Autodesk Inventor part; units mm, degrees
ref_plane "Start plane" through (0, 0, 0) normal (0, 0, 1) x (1, 0, 0)
ref_plane "End plane" through (0, 0, 796) normal (0, 0, 1) x (1, 0, 0)
ref_plane "YZ Plane" through (0, 0, 0) normal (1, 0, 0) x (0, 1, 0)
ref_plane "Start plane" through (0, 0, 0) normal (0, 0, 1) x (1, 0, 0)
ref_plane "End plane" through (0, 0, 796) normal (0, 0, 1) x (1, 0, 0)
sketch "Sketch" plane through (0, 0, 0) normal (0, 0, 1) x (1, 0, 0)
  line L0 (-10, -16) -> (-10, 16)
  line L1 (-6, 20) -> (6, 20)
  line L2 (10, 16) -> (10, -16)
  line L3 (6, -20) -> (-6, -20)
  arc A0 (-10, -16) -> (-6, -20) centre (-6, -16) ccw
  arc A1 (10, 16) -> (6, 20) centre (6, 16) ccw
  arc A2 (-6, 20) -> (-10, 16) centre (-6, 16) ccw
  arc A3 (6, -20) -> (10, -16) centre (6, -16) ccw
  arc A4 (-6, 18) -> (-8, 16) centre (-6, 16) ccw
  line L4 (-6, 18) -> (6, 18)
  arc A5 (8, 16) -> (6, 18) centre (6, 16) ccw
  line L5 (8, 16) -> (8, -16)
  arc A6 (6, -18) -> (8, -16) centre (6, -16) ccw
  line L6 (6, -18) -> (-6, -18)
  arc A7 (-8, -16) -> (-6, -18) centre (-6, -16) ccw
  line L7 (-8, -16) -> (-8, 16)
  line L8 (0, 29.1598) -> (0, -29.1598) construction
  line L9 (-15.1598, 0) -> (15.1598, 0) construction
  dimension "d7" = 4
  dimension "d9" = 20
  dimension "d11" = 40
  dimension "d12" = 2
  dimension "d15" = 10
  dimension "d16" = 20
extrude "Body" add sketch "Sketch" along normal up to surface (796 mm away) from surface at 0
sketch "Sketch3" plane through (0, 0, 0) normal (0, 0, 1) x (1, 0, 0)
  line L0 (0, 0) -> (10, 0)
ref_plane "Work Plane3" through (0, 0, 0) normal (0, -1, 0) x (1, 0, 0)
sketch "Sketch5" plane through (-6, -20, 0) normal (0, -1, 0) x (1, 0, 0)
  line L0 (-4, 0) -> (-4, 796)
  line L1 (-4, 796) -> (0, 796)
  line L2 (12, 796) -> (0, 796)
  line L3 (12, 796) -> (16, 796)
  line L4 (16, 0) -> (16, 796)
  line L5 (16, 796) -> (-4, 782.7623)
  point P0 (6, 0)
  dimension "d19" = 33.5
extrude "Extrusion2" cut sketch "Sketch5" against normal through all
sketch "Sketch4" plane through (0, 0, 0) normal (0, -1, 0) x (1, 0, 0)
  line L0 (-2, 0) -> (12, 0)
  line L1 (-2, 796) -> (12, 796)
  dimension "d18" = 796
equation "\"d7\" = G_IR"
equation "\"d9\" = G_W"
equation "\"d11\" = G_H"
equation "\"d12\" = G_T"
equation "\"d15\" = 0.5 * d9"
equation "\"d16\" = 0.5 * d11"
equation "\"d3\" = G_L"
equation "\"G_W\" = 20"
equation "\"G_H\" = 40"
equation "\"G_T\" = 2"
equation "\"G_IR\" = 4"
equation "\"G_L\" = d18"
equation "\"G_OFFSET_START\" = 0"
equation "\"G_OFFSET_END\" = 0"
equation "\"d14\" = G_OFFSET_END + B_L"
equation "\"B_L\" = 796"
properties part number "ISO 4019 - 40x20x2 - 796" material "Steel, Mild"
The listing builds one solid part. Answer for the finished solid, in the listing's coordinates (mm). A direction names the side the tool comes from. Give positions to 0.01 mm unless a question says otherwise; leave off trailing zeros. Write each loop counter-clockwise with the first axis right and the second up, starting at its lowest first coordinate (ties: lowest second). Pieces come first, ordered by that corner, then holes.
Item 1: Section A-A, the plane y = -6.5 is taken. Write down the section's boundary in (x, z).
Item 2: Determine the mould class of faces 1 (the flat face through (0, 20, 391)), 2 (the flat face through (0, -18, 391)), 3 (the flat face through (8.195, -0.093, 794.805)) for opening direction X: released by +X, released by -X, zero draft, split by the parting line, or undercut.
Item 3: Which of the six approach directions +Z, -Z, +X, -X, +Y, -Y give full straight-line access (tool end or side, diameter ignored) to faces 4 (the flat face through (-8.2, 0.1, 0)), 5 (the flat face through (8, 0, 392))?
Item 4: Section C-C, the plane x = 1 is taken. Write down the section's boundary in (y, z), plus the area to 3 significant figures.
Item 5: Find the intervals of material crossed by line 1 along X through (y, z) = (-7, 365); line 2 along X through (y, z) = (16.5, 547); line 3 along Y through (x, z) = (-1.25, 756), in increasing order.
Item 6: Section B-B, the plane z = 629.5 is taken. Write down the section's boundary in (x, y).
Completed:
1. outline: (-10, 0) - (-8, 0) - (-8, 784.09) - (-10, 782.76) - close; (8, 0) - (10, 0) - (10, 796) - (8, 794.68) - close
2. face 1: zero draft
2. face 2: undercut
2. face 3: released by -X
3. face 4: -Z, +X, -X, +Y, -Y
3. face 5: +Z, -Z
4. outline: (-20, 0) - (-18, 0) - (-18, 790.04) - (-20, 790.04) - close; (18, 0) - (20, 0) - (20, 790.04) - (18, 790.04) - close
4. area: 3,160 mm2
5. line 1: x = -10 to -8, 8 to 10
5. line 2: x = -9.97 to -7.94, 7.94 to 9.97
5. line 3: y = -20 to -18, 18 to 20
6. outline: (-10, -16) arc R4 ccw to (-6, -20) - (6, -20) arc R4 ccw to (10, -16) - (10, 16) arc R4 ccw to (6, 20) - (-6, 20) arc R4 ccw to (-10, 16) - close; hole (-8, -16) arc R2 ccw to (-6, -18) - (6, -18) arc R2 ccw to (8, -16) - (8, 16) arc R2 ccw to (6, 18) - (-6, 18) arc R2 ccw to (-8, 16) - close
